Verification items for the finished model (mm, model axes). Face numbers are marked on the shaded views. A direction names the side the tool comes from. Round coordinates to 2 decimals unless told otherwise and drop trailing zeros. Write each loop counter-clockwise with the first axis right and the second up, starting at its lowest first coordinate (ties: lowest second). Pieces come first, ordered by that corner, then holes.
from build123d import *

# Parameters (mm, degrees)
AUFSATZ_LINEAR_AUSTRAGEN1_DEPTH = 16
SCHNITT_LINEAR_AUSTRAGEN1_DEPTH = 16
VERRUNDUNG3_R                   = 3
SKIZZE6_R                       = 1.9
SCHNITT_LINEAR_AUSTRAGEN2_DEPTH = 4.5
KREISMUSTER1_COUNT              = 3
FASE1_SIZE                      = 0.5


with BuildPart() as part:
    # Skizze3 → Aufsatz-Linear austragen1 (new body)
    with BuildSketch(Plane.XY):
        with BuildLine():
            ThreePointArc((3.545052466, -3.382691682), (4.66017693, -1.514183272), (4.856303974, 0.652925499))
            ThreePointArc((4.856303974, 0.652925499), (4.802835407, 1.560535822), (4.312612425, 2.326236032))
            ThreePointArc((4.312612425, 2.326236032), (2.880147736, 3.964183272), (0.879711407, 4.820384615))
            ThreePointArc((0.879711407, 4.820384615), (0, 5.05), (-0.879711407, 4.820384615))
            ThreePointArc((-0.879711407, 4.820384615), (-2.880147736, 3.964183272), (-4.312612425, 2.326236032))
            ThreePointArc((-4.312612425, 2.326236032), (-4.802835407, 1.560535822), (-4.856303974, 0.652925499))
            ThreePointArc((-4.856303974, 0.652925499), (-4.66017693, -1.514183272), (-3.545052466, -3.382691682))
            ThreePointArc((-3.545052466, -3.382691682), (-2.968315524, -4.085535822), (-2.121649509, -4.416854465))
            ThreePointArc((-2.121649509, -4.416854465), (0, -4.9), (2.121649509, -4.416854465))
            ThreePointArc((2.121649509, -4.416854465), (2.968315524, -4.085535822), (3.545052466, -3.382691682))
        make_face()
    extrude(amount=AUFSATZ_LINEAR_AUSTRAGEN1_DEPTH)

    # Skizze4 → Schnitt-Linear austragen1 (cut)
    with BuildSketch(Plane(origin=(0, 0, 0), x_dir=(-1, 0, 0), z_dir=(0, 0, -1))):
        with BuildLine():
            Line((-1.532970972, 2.1), (1.532970972, 2.1))
            ThreePointArc((1.532970972, 2.1), (0, -2.6), (-1.532970972, 2.1))
        make_face()
    extrude(amount=-SCHNITT_LINEAR_AUSTRAGEN1_DEPTH, mode=Mode.SUBTRACT)

    # Skizze5 → Rotation1 (revolve)
    with BuildSketch(Plane(origin=(0, 0, 0), x_dir=(1, 0, 0), z_dir=(0, 1, 0)), mode=Mode.PRIVATE) as rotation1_sk:
        Polygon((-4.890933678, -16), (-16.890933678, -16), (-16.890933678, -11), (-6.890933678, -11), (-6.890933678, -8), (-4.890933678, -8), align=None)
    revolve(rotation1_sk.sketch.rotate(Axis((0, 0, 16), (0, 0, -1)), 180), axis=Axis((0, 0, 16), (0, 0, -1)))

    # Verrundung3
    verrundung3_edges = [part.edges().sort_by_distance(p)[0] for p in [
        (-16.890933678, 0, 11),
    ]]
    fillet(verrundung3_edges, radius=VERRUNDUNG3_R)

    # Skizze6 → Schnitt-Linear austragen2 (cut)
    with BuildSketch(Plane.XY.offset(16)):
        with Locations((0, 12)):
            Circle(SKIZZE6_R)
    schnitt_linear_austragen2 = extrude(amount=-SCHNITT_LINEAR_AUSTRAGEN2_DEPTH, mode=Mode.SUBTRACT)

    # Kreismuster1: Schnitt-Linear austragen2 ×3 about axis
    kreismuster1_axis = Axis((0, 0, 0), (0, 0, 1))
    for i in range(1, KREISMUSTER1_COUNT):
        add(schnitt_linear_austragen2.rotate(kreismuster1_axis, i * 360 / KREISMUSTER1_COUNT), mode=Mode.SUBTRACT)

    # Fase1
    fase1_edges = [part.edges().sort_by_distance(p)[0] for p in [
        (0, 5.05, 0),
        (2.880147736, 3.964183272, 0),
        (4.802835407, 1.560535822, 0),
        (4.66017693, -1.514183272, 0),
        (2.968315524, -4.085535822, 0),
        (0, -4.9, 0),
        (-2.968315524, -4.085535822, 0),
        (-4.66017693, -1.514183272, 0),
        (-4.802835407, 1.560535822, 0),
        (-2.880147736, 3.964183272, 0),
    ]]
    chamfer(fase1_edges, length=FASE1_SIZE)


solid = part.part
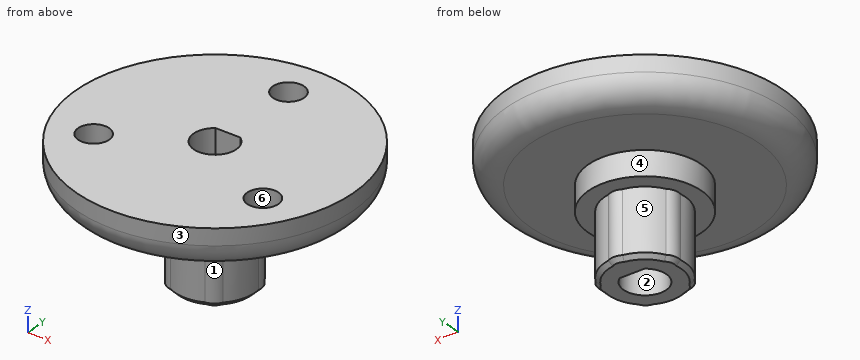
Q1. Sectioned sample at C-C (z = 10). Enter the section's corners in (x, y), plus the area to 3 significant figures.
Recorded:
outline: circle Ø13.78 at (0, 0); hole (-1.53, 2.1) arc R2.6 ccw (long way) to (1.53, 2.1) - close
area: 129 mm2
Q2. Tool access check on the marked faces 4, 5 and 6. Record the directions out of +Z, -Z, +X, -X, +Y, -Y that give a thin tool (end or side, any length) a straight path to the whole face; none if there is none.
Recorded:
face 4: -Z
face 5: -Z, -X, +Y
face 6: +Z
Q3. Sectioned sample at B-B (z = 13.25). Enter the section's corners in (x, y), plus the area to 3 significant figures.
Recorded:
outline: circle Ø33.59 at (0, 0); hole circle Ø3.8 at (-10.39, -6); hole circle Ø3.8 at (0, 12); hole (-1.53, 2.1) arc R2.6 ccw (long way) to (1.53, 2.1) - close; hole circle Ø3.8 at (10.39, -6)
area: 832 mm2
Q4. Material ranges on line 1 along Y through (x, z) = (0, 12.65); line 2 along Z through (x, y) = (-12, 2); line 3 along Y through (x, z) = (0, 9.5), recorded low to high.
Recorded:
line 1: y = -16.57 to -2.6, 2.1 to 10.1, 13.9 to 16.57
line 2: z = 11 to 16
line 3: y = -6.89 to -2.6, 2.1 to 6.89
Q5. Sectioned sample at D-D (z = 5). Enter the section's corners in (x, y), plus the area to 3 significant figures.
Recorded:
outline: (-4.86, 0.65) arc R4.9 ccw to (-3.55, -3.38) arc R1.8 ccw to (-2.12, -4.42) arc R4.9 ccw to (2.12, -4.42) arc R1.8 ccw to (3.55, -3.38) arc R4.9 ccw to (4.86, 0.65) arc R1.8 ccw to (4.31, 2.33) arc R4.9 ccw to (0.88, 4.82) arc R1.8 ccw to (-0.88, 4.82) arc R4.9 ccw to (-4.31, 2.33) arc R1.8 ccw to start; hole (-1.53, 2.1) arc R2.6 ccw (long way) to (1.53, 2.1) - close
area: 56.1 mm2
Q6. Sectioned sample at A-A (y = 0). Enter the section's corners in (x, z).
Recorded:
outline: (-16.89, 14) arc R3 ccw to (-13.89, 11) - (-6.89, 11) - (-6.89, 8) - (-4.9, 8) - (-4.9, 0.5) - (-4.4, 0) - (-2.6, 0) - (-2.6, 16) - (-16.89, 16) - close; (2.6, 0) - (4.4, 0) - (4.9, 0.5) - (4.9, 8) - (6.89, 8) - (6.89, 11) - (13.89, 11) arc R3 ccw to (16.89, 14) - (16.89, 16) - (2.6, 16) - close
Q7. Depth check by flat-ended pin: P1, Ø1, axis at y = 3, z = 6, coming from the +X side; P2, Ø3, axis at x = -11.5, y = -9, coming from the -Z side; P3, Ø1.9, axis at x = 0, y = 11.5, coming from the +Z side; P4, Ø3, axis at y = -7, z = 2.5, coming from the -X side. Enter the tip coordinate at first touch or a pass-through.
Recorded:
P1: stops at x = 4.21
P2: stops at z = 11
P3: stops at z = 11.5
P4: passes through
Q8. Release check for a two-part mould opening along X. For the marked faces 1, 2 and 3 record: released by +X, released by -X, zero draft, split by the parting line, or undercut.
Recorded:
face 1: released by +X
face 2: undercut
face 3: split by the parting line
